Design review of the part built by this model. Coordinates are the model's own, in mm. A direction names the side the tool comes from. Coordinates: 2 decimals unless noted, no trailing zeros. Loops run counter-clockwise (first coordinate to the right, second up) from the corner with the lowest first, then second, coordinate; pieces in that order, holes last. Notation, with made-up numbers: (73, -39.75) -> (92, -39.75) arc R15 cw to (92, -20.75) -> close; hole circle Ø9 at (78, 84.5). An arc over 180 degrees is marked (long way). Answer in a Markdown table with one row per item.
```python
from build123d import *

# Parameters (mm, degrees)
PAD_DEPTH        = 4
HOLE_D           = 3
HOLE_CSINK_D     = 7
HOLE_CSINK_ANGLE = 90
SKETCH002_R      = 45
PAD001_DEPTH     = 10
SKETCH003_R      = 43.8
POCKET_DEPTH     = 14.001
SKETCH004_R      = 2.25
HOLE001_DEPTH    = 25
CHAMFER_SIZE     = 1


with BuildPart() as part:
    # Sketch → Pad (new body)
    with BuildSketch(Plane.XY):
        with BuildLine():
            Line((-52.5, 46.5), (-52.5, -46.5))
            ThreePointArc((-52.5, -46.5), (-50.742641, -50.742641), (-46.5, -52.5))
            Line((-46.5, -52.5), (46.5, -52.5))
            ThreePointArc((46.5, -52.5), (50.742641, -50.742641), (52.5, -46.5))
            Line((52.5, -46.5), (52.5, 46.5))
            ThreePointArc((52.5, 46.5), (50.742641, 50.742641), (46.5, 52.5))
            Line((46.5, 52.5), (-46.5, 52.5))
            ThreePointArc((-46.5, 52.5), (-50.742641, 50.742641), (-52.5, 46.5))
        make_face()
    extrude(amount=PAD_DEPTH)

    # Hole (through all)
    with Locations(Plane(origin=(0, 0, 0), x_dir=(1, 0, 0), z_dir=(0, 0, -1))):
        with Locations((-47, -47), (47, -47), (47, 47), (-47, 47)):
            CounterSinkHole(HOLE_D / 2, HOLE_CSINK_D / 2, counter_sink_angle=HOLE_CSINK_ANGLE)

    # Sketch002 (on DatumPlane) → Pad001 (join)
    with BuildSketch(Plane.XY.offset(4)):
        Circle(SKETCH002_R)
    extrude(amount=PAD001_DEPTH)

    # Sketch003 (on Face20 of Pad001) → Pocket (cut, through all)
    with BuildSketch(Plane.XY.offset(14)):
        Circle(SKETCH003_R)
    extrude(amount=-POCKET_DEPTH, mode=Mode.SUBTRACT)

    # Sketch004 → Hole001 (cut)
    with BuildSketch(Plane.XY):
        with Locations((0, 48)):
            Circle(SKETCH004_R)
        with Locations((48, 0)):
            Circle(SKETCH004_R)
        with Locations((0, -48)):
            Circle(SKETCH004_R)
        with Locations((-48, 0)):
            Circle(SKETCH004_R)
    extrude(amount=HOLE001_DEPTH, mode=Mode.SUBTRACT)

    # Chamfer
    chamfer_edges = [part.edges().sort_by_distance(p)[0] for p in [
        (-52.5, 0, 0),
    ]]
    chamfer(chamfer_edges, length=CHAMFER_SIZE)


solid = part.part
```
(1) To check wall thickness, follow probe 1 along Y at (x, z) = (0, 2.65); probe 2 along X at (y, z) = (-47, 3.55); probe 3 along Y at (x, z) = (48, 2.05). State the ranges of each line that lie inside material, in increasing order.
Evaluation:
| item | result |
|---|---|
| probe 1 | y = -52.5 to -50.25, -45.75 to -43.8, 43.8 to 45.75, 50.25 to 52.5 |
| probe 2 | x = -52.48 to -48.5, -45.5 to -2.02, 2.02 to 45.5, 48.5 to 52.48 |
| probe 3 | y = -52.31 to -48.12, -45.88 to -2.25, 2.25 to 45.88, 48.12 to 52.31 |
(2) Draft analysis for pull direction Y (two halves, no side actions). For faces 3 (the cylindrical face through (-34.76, -26.65, 7.1)), 4 (the cylindrical face through (20.765, -39.923, 8.93)), 5 (the conical face through (50.268, 50.186, 0.271)), state which applies: pulls with the +Y half, pulls with the -Y half, needs draft (parallel to the pull), parting line crosses it, or undercut.
Evaluation:
| item | result |
|---|---|
| face 3 | undercut |
| face 4 | parting line crosses it |
| face 5 | pulls with the +Y half |
(3) For pin 1 (5 mm diameter, centred on x = 48, y = 0, fed in from -Z); pin 2 (6 mm diameter, centred on x = 14, y = 35.5, fed in from +Z); pin 3 (1.5 mm diameter, centred on x = -10, z = 7, fed in from -Y); pin 4 (5 mm diameter, centred on x = 47, y = -47, fed in from -Z), all flat-tipped, find the tip position at first contact; note any pin that passes through.
Evaluation:
| item | result |
|---|---|
| pin 1 | stops at z = 0 |
| pin 2 | passes through |
| pin 3 | stops at y = -44.04 |
| pin 4 | stops at z = 1 |
(4) Take a section at C-C on y = 29.5. Give the boundary of the cut face in (x, z).
Evaluation:
| item | result |
|---|---|
| outline | (-52.5, 1) -> (-51.5, 0) -> (-32.38, 0) -> (-32.38, 14) -> (-33.98, 14) -> (-33.98, 4) -> (-52.5, 4) -> close; (32.38, 0) -> (51.5, 0) -> (52.5, 1) -> (52.5, 4) -> (33.98, 4) -> (33.98, 14) -> (32.38, 14) -> close |
(5) Tool access review of faces 1 (the flat face through (23, -39, 4)), 2 (the cylindrical face through (-50.789, -50.696, 2.479)): name each direction out of +Z, -Z, +X, -X, +Y, -Y from which nothing blocks a thin tool from reaching the whole face with its end or side.
Evaluation:
| item | result |
|---|---|
| face 1 | +Z |
| face 2 | +Z, -Z, -X, -Y |
(6) Take a section at A-A on x = 0. Give the boundary of the cut face in (y, z).
Evaluation:
| item | result |
|---|---|
| outline | (-52.5, 1) -> (-51.5, 0) -> (-50.25, 0) -> (-50.25, 4) -> (-52.5, 4) -> close; (-45.75, 0) -> (-43.8, 0) -> (-43.8, 14) -> (-45, 14) -> (-45, 4) -> (-45.75, 4) -> close; (43.8, 0) -> (45.75, 0) -> (45.75, 4) -> (45, 4) -> (45, 14) -> (43.8, 14) -> close; (50.25, 0) -> (51.5, 0) -> (52.5, 1) -> (52.5, 4) -> (50.25, 4) -> close |
(7) Take a section at D-D on x = -29. Give the boundary of the cut face in (y, z).
Evaluation:
| item | result |
|---|---|
| outline | (-52.5, 1) -> (-51.5, 0) -> (-32.82, 0) -> (-32.82, 14) -> (-34.41, 14) -> (-34.41, 4) -> (-52.5, 4) -> close; (32.82, 0) -> (51.5, 0) -> (52.5, 1) -> (52.5, 4) -> (34.41, 4) -> (34.41, 14) -> (32.82, 14) -> close |
